Here's how the part is built. I have some questions about the finished solid (model axes, mm). A direction names the side the tool comes from. Give positions to 0.01 mm unless a question says otherwise; leave off trailing zeros. Loops run counter-clockwise (first coordinate to the right, second up) from the corner with the lowest first, then second, coordinate; pieces in that order, holes last.
Q1. Suppose I cut it at D-D (y = 7.75). List the corners of the cut face in (x, z) for me.
Q2. Suppose I cut it at C-C (x = -9.25). List the corners of the cut face in (y, z) for me, and give its area (3 significant figures).
Q3. I'm going to push flat-ended pins straight in: P1, Ø5, axis at x = 8, y = 5.5, coming from the +Z side; P2, Ø1, axis at y = 5.5, z = 4, coming from the -X side; P3, Ø1.4, axis at x = 0, z = 2.5, coming from the -Y side; P4, Ø3, axis at y = 6, z = 1.5, coming from the -X side. Where does each tip first touch, or does it pass through?
Q4. Thinking about a two-plate mould opening in X: for faces 1 (the face through (0, 2, 5)), 2 (the face through (5.1, 4.42, 2.46)), 3 (the face through (-13, 2, 2)), 4 (the face through (-0.03, 1.3, 3.25)), which applies, pulls with the +X half, pulls with the -X half, needs draft (parallel to the pull), parting line crosses it, or undercut?
Q5. I need wall thicknesses on probe 1 along X at (y, z) = (1.05, 2.5); probe 2 along Z at (x, y) = (8.5, 1); probe 3 along X at (y, z) = (3.5, 3.4). Which ranges of each line are inside material? Lowest first, please.
Q6. Suppose I cut it at B-B (z = 2.15). List the corners of the cut face in (x, y) for me, and give its area (3 significant figures).
Q7. Suppose I cut it at A-A (y = 3). List the corners of the cut face in (x, z) for me, and give its area (3 significant figures).
Q8. For faces 5 (the face through (0, 2, 0)), 6 (the face through (-11.1, 4, 1.9)), 7 (the face through (10.5, 4, 2.5)), which set-ups out of +Z, -Z, +X, -X, +Y, -Y let a thin tool reach every point of the face, with its end or its side?
```python
from build123d import *
from build123d.topology import SkipClean

# Parameters (mm, degrees)
BOSS_EXTRUDE1_DEPTH     = 5
SKETCH2_R               = 1.5
CUT_EXTRUDE1_DEPTH      = 5
CUT_EXTRUDE2_DEPTH      = 15.798648587
CUT_EXTRUDE2_DEPTH_BACK = 15.798648587
SKETCH3_R               = 0.75


with BuildPart() as part:
    # Sketch1 → Boss-Extrude1 (new body)
    with BuildSketch(Plane.XY):
        with BuildLine():
            Line((-13, 0), (0, 0))
            Line((0, 0), (0, 2.5))
            ThreePointArc((0, 2.5), (-2, 4.5), (0, 6.5))
            Line((0, 6.5), (0, 9))
            ThreePointArc((0, 9), (-2.790781528, 8.030090432), (-4.378538299, 5.538461538))
            ThreePointArc((-4.378538299, 5.538461538), (-5.084207974, 4.431070919), (-6.32455532, 4))
            Line((-6.32455532, 4), (-13, 4))
            Line((-13, 4), (-13, 0))
        make_face()
        with BuildLine():
            Line((0, 2.5), (0, 0))
            Line((0, 0), (13, 0))
            Line((13, 0), (13, 4))
            Line((13, 4), (6.32455532, 4))
            ThreePointArc((6.32455532, 4), (5.084207974, 4.431070919), (4.378538299, 5.538461538))
            ThreePointArc((4.378538299, 5.538461538), (2.790781528, 8.030090432), (0, 9))
            Line((0, 9), (0, 6.5))
            ThreePointArc((0, 6.5), (1.414213562, 5.914213562), (2, 4.5))
            ThreePointArc((2, 4.5), (1.414213562, 3.085786438), (0, 2.5))
        make_face()
    extrude(amount=BOSS_EXTRUDE1_DEPTH)

    # Sketch2 → Cut-Extrude1 (cut)
    with BuildSketch(Plane(origin=(0, 4, 0), x_dir=(1, 0, 0), z_dir=(0, 1, 0))):
        with Locations(Location((-9.517345142, -2.5, 0), (0, 0, 270))):
            Circle(SKETCH2_R)
        with Locations(Location((8.482654858, -2.5, 0), (0, 0, 270))):
            Circle(SKETCH2_R)
    extrude(amount=-CUT_EXTRUDE1_DEPTH, mode=Mode.SUBTRACT)

    # Sketch3 → Cut-Extrude2 (cut, two sides: drawn at the far end of the back side and taken through both)
    with SkipClean():  # the faces are left unmerged after this step: merging them gives an invalid solid
        with BuildSketch(Plane(origin=(0, 4, 0), x_dir=(1, 0, 0), z_dir=(0, 1, 0)).offset(-CUT_EXTRUDE2_DEPTH_BACK)):
            with Locations(Location((0, -2.5, 0), (0, 0, 90))):
                Circle(SKETCH3_R)
        extrude(amount=CUT_EXTRUDE2_DEPTH + CUT_EXTRUDE2_DEPTH_BACK, mode=Mode.SUBTRACT)


solid = part.part
```
Solutions:
1. outline: (-3.11, 0) - (3.11, 0) - (3.11, 5) - (-3.11, 5) - close; hole circle Ø1.5 at (0, 2.5)
2. outline: (0, 0) - (4, 0) - (4, 1.02) - (0, 1.02) - close; (0, 3.98) - (4, 3.98) - (4, 5) - (0, 5) - close
2. area: 8.19 mm2
3. P1: stops at z = 5
3. P2: stops at x = -4.59
3. P3: passes through
3. P4: stops at x = -5
4. face 1: needs draft
4. face 2: pulls with the +X half
4. face 3: pulls with the -X half
4. face 4: undercut
5. probe 1: x = -13 to -11.02, -8.02 to -0.75, 0.75 to 6.98, 9.98 to 13
5. probe 2: z = 0 to 1, 4 to 5
5. probe 3: x = -13 to -10.72, -8.32 to -1.73, 1.73 to 7.28, 9.68 to 13
6. outline: (-13, 0) - (-10.98, 0) - (-10.98, 4) - (-13, 4) - close; (-8.06, 0) - (-0.66, 0) - (-0.66, 2.61) arc R2 cw to (-0.66, 6.39) - (-0.66, 8.95) arc R4.5 ccw to (-4.38, 5.54) arc R2 cw to (-6.32, 4) - (-8.06, 4) - close; (0.66, 0) - (7.02, 0) - (7.02, 4) - (6.32, 4) arc R2 cw to (4.38, 5.54) arc R4.5 ccw to (0.66, 8.95) - (0.66, 6.39) arc R2 cw to (0.66, 2.61) - close; (9.94, 0) - (13, 0) - (13, 4) - (9.94, 4) - close
6. area: 98.9 mm2
7. outline: (-13, 0) - (-1.32, 0) - (-1.32, 5) - (-13, 5) - close; (1.32, 0) - (13, 0) - (13, 5) - (1.32, 5) - close; hole circle Ø3 at (-9.52, 2.5); hole circle Ø3 at (8.48, 2.5)
7. area: 103 mm2
8. face 5: -Z, +X, -X, +Y, -Y
8. face 6: +Z, -Z, -X, +Y
8. face 7: +Z, -Z, +X, +Y
